Design review of the part built by this model. Coordinates are the model's own, in mm. A direction names the side the tool comes from. Coordinates: 2 decimals unless noted, no trailing zeros. Write each loop counter-clockwise with the first axis right and the second up, starting at its lowest first coordinate (ties: lowest second). Pieces come first, ordered by that corner, then holes. Notation, with made-up numbers: (-40, 71) - (16, 71) arc R20 cw to (16, 107) - close; hole circle Ø11 at (29, 49). An arc over 180 degrees is marked (long way). Answer as a JSON object with one key per item and string values.
```python
from build123d import *

# Parameters (mm, degrees)
BASE_EXTRUSION_DEPTH                     = 279.4
BASE_T_SLOT_DEPTH                        = 283.823092451
BASE_TABS_DEPTH                          = 6.35
SKETCH5_W                                = 40.64
SKETCH5_H                                = 20.066
SERVO_SLOT_DEPTH                         = 283.823092451
SKETCH6_R                                = 1.778
SERVO_MOUNTING_HOLES_DEPTH               = 283.823092451
FILLER_EXTRUSION_TO_FUNNEL_SUPPORT_DEPTH = 279.4
SIDE_T_SLOT_DEPTH                        = 284.874808603
SKETCH9_W                                = 6.35
SKETCH9_H                                = 12.7
SIDE_TABS_DEPTH                          = 6.35


with BuildPart() as part:
    # Sketch2 → Base Extrusion (new body)
    with BuildSketch(Plane.XY):
        Polygon((-71.1004567, -13.712301035), (-75.59058476, -18.202429096), (-47.146344636, -46.64666922), (-42.656216575, -42.15654116), align=None)
    extrude(amount=BASE_EXTRUSION_DEPTH)

    # Sketch3 → Base T Slot (cut, through all)
    with BuildSketch(Plane(origin=(-46.896506928, -46.896506928, 0), x_dir=(0, 0, 1), z_dir=(-0.7071067811865479, -0.7071067811865472, 0))):
        Polygon((0, 22.600038952), (0, 18.332838952), (8.763, 18.332838952), (8.763, 16.021438952), (11.938, 16.021438952), (11.938, 18.332838952), (15.24, 18.332838952), (15.24, 22.600038952), (11.938, 22.600038952), (11.938, 24.911438952), (8.763, 24.911438952), (8.763, 22.600038952), align=None)
    extrude(amount=-BASE_T_SLOT_DEPTH, mode=Mode.SUBTRACT)

    # Sketch4 → Base Tabs (add)
    with BuildSketch(Plane(origin=(0, 0, 0), x_dir=(-1, 0, 0), z_dir=(0, 0, -1))):
        Polygon((75.59058476, -18.202429096), (65.858592758, -27.934421097), (61.368464698, -23.444293037), (71.1004567, -13.712301035), align=None)
        Polygon((42.656216575, -42.15654116), (52.388208577, -32.424549158), (56.878336637, -36.914677218), (47.146344636, -46.64666922), align=None)
    extrude(amount=BASE_TABS_DEPTH)

    # Sketch5 → Servo Slot (cut, through all)
    with BuildSketch(Plane(origin=(-42.406378867, -42.406378867, 0), x_dir=(0, 0, -1), z_dir=(0.7071067811865476, 0.7071067811865476, 0))):
        with Locations((-246.38, 34.529271287)):
            Rectangle(SKETCH5_W, SKETCH5_H)
    extrude(amount=-SERVO_SLOT_DEPTH, mode=Mode.SUBTRACT)

    # Sketch6 → Servo Mounting Holes (cut, through all)
    with BuildSketch(Plane(origin=(-42.406378867, -42.406378867, 0), x_dir=(0, 0, -1), z_dir=(0.7071067811865476, 0.7071067811865476, 0))):
        with Locations((-270.88, 39.529271287)):
            Circle(SKETCH6_R)
        with Locations(Location((-270.88, 25.54655403, 0), (0, 0, 90))):
            Circle(SKETCH6_R)
        with Locations((-221.88, 39.529271287)):
            Circle(SKETCH6_R)
        with Locations(Location((-221.88, 25.54655403, 0), (0, 0, 90))):
            Circle(SKETCH6_R)
    extrude(amount=-SERVO_MOUNTING_HOLES_DEPTH, mode=Mode.SUBTRACT)

    # Sketch7 → Filler Extrusion to Funnel Support (add)
    with BuildSketch(Plane.XY.offset(279.4)):
        Polygon((-47.146344636, -46.64666922), (-42.656216575, -42.15654116), (-38.166088515, -46.64666922), (-42.656216575, -51.136797281), align=None)
        Polygon((-75.59058476, -18.202429096), (-71.1004567, -13.712301035), (-75.59058476, -9.222172974), (-80.080712821, -13.712301035), align=None)
    extrude(amount=-FILLER_EXTRUSION_TO_FUNNEL_SUPPORT_DEPTH)

    # Sketch8 → Side T Slot (cut, through all)
    with BuildSketch(Plane(origin=(-42.406378867, -42.406378867, 0), x_dir=(0.7071067811865477, -0.7071067811865474, 0), z_dir=(0.7071067811865474, 0.7071067811865477, 0))):
        Polygon((5.996676125, -136.7536), (5.996676125, -132.4864), (-2.766323875, -132.4864), (-2.766323875, -130.175), (-5.941323875, -130.175), (-5.941323875, -132.4864), (-9.243323875, -132.4864), (-9.243323875, -136.7536), (-5.941323875, -136.7536), (-5.941323875, -139.065), (-2.766323875, -139.065), (-2.766323875, -136.7536), align=None)
    extrude(amount=-SIDE_T_SLOT_DEPTH, mode=Mode.SUBTRACT)

    # Sketch9 → Side Tabs (add)
    with BuildSketch(Plane(origin=(4.240290353, -4.240290353, 0), x_dir=(-0.7071067811865475, -0.7071067811865477, 0), z_dir=(0.7071067811865477, -0.7071067811865475, 0))):
        with Locations((63.146676125, -206.375)):
            Rectangle(SKETCH9_W, SKETCH9_H)
        with Locations((63.146676125, -155.575)):
            Rectangle(SKETCH9_W, SKETCH9_H)
    extrude(amount=SIDE_TABS_DEPTH)


solid = part.part
```
(1) Take a section at B-B, the plane z = 35. Write out the cut boundary in (x, y).
Solved:
{"outline": "(-80.08, -13.71) - (-42.66, -51.14) - (-38.17, -46.65) - (-75.59, -9.22) - close"}
(2) Take a section at C-C, the plane z = 156.5. Write out the cut boundary in (x, y).
Solved:
{"outline": "(-80.08, -13.71) - (-38.17, -55.63) - (-33.68, -51.14) - (-75.59, -9.22) - close"}
(3) For pin 1 (17.5 mm diameter, centred on x = -65.5, y = -18, fed in from +Z); pin 2 (6 mm diameter, centred on x = -52, z = 168.5, fed in from -Y); pin 3 (6.5 mm diameter, centred on x = -61, y = -28.5, fed in from -Z); pin 4 (7 mm diameter, centred on x = -37.5, y = -52.5, fed in from -Z) (3 decimals), all flat-tipped, find the tip position at first contact; note any pin that passes through.
Solved:
{"pin 1": "stops at z = 279.4", "pin 2": "stops at y = -44.79", "pin 3": "stops at z = 0", "pin 4": "stops at z = 149.225"}
(4) Tool access review of faces 4 (the face through (-59, -30, 15.24)), 5 (the face through (-51.156, -38.084, 134.59)), 6 (the face through (-48, -42, 139.065)): name each direction out of +Z, -Z, +X, -X, +Y, -Y from which nothing blocks a thin tool from reaching the whole face with its end or side.
Solved:
{"face 4": "-Z", "face 5": "+X, -Y", "face 6": "none"}
(5) Take a section at A-A, the plane z = 243. Write out the cut boundary in (x, y), and give its area (3 significant figures).
Solved:
{"outline": "(-80.08, -13.71) - (-75.59, -18.2) - (-71.1, -13.71) - (-75.59, -9.22) - close; (-64.22, -29.58) - (-42.66, -51.14) - (-38.17, -46.65) - (-59.73, -25.08) - close", "area": "234 mm^2"}
(6) To check wall thickness, follow line 1 (Z direction, x = -76.5, y = -14); line 2 (Y direction, x = -54.5, z = 160.5); line 3 (X direction, y = -50, z = 229). State the ranges of each line that lie inside material, in increasing order. Write a range as from..to.
Solved:
{"line 1": "z = 0..279.4", "line 2": "y = -39.29..-30.31", "line 3": "x = -43.79..-41.52"}
(7) The part is to be moulded in two halves that separate along X. For faces 1 (the face through (-40.38, -48.86, 246.53)), 2 (the face through (-46.576, -42.664, 137.925)), 3 (the face through (-50, -39, 136.754)), say which applies: pulls with the +X half, pulls with the -X half, needs draft (parallel to the pull), parting line crosses it, or undercut.
Solved:
{"face 1": "pulls with the +X half", "face 2": "undercut", "face 3": "needs draft"}
